Verification items for the finished model (mm, model axes). Face numbers are marked on the shaded views. A direction names the side the tool comes from. Coordinates: 2 decimals unless noted, no trailing zeros. Loops run counter-clockwise (first coordinate to the right, second up) from the corner with the lowest first, then second, coordinate; pieces in that order, holes last. Notation, with made-up numbers: (-13, 58.5) -> (-7, 58.5) arc R29 cw to (-7, 92.5) -> close; hole circle Ø3 at (41, 7.5). An arc over 180 degrees is marked (long way). Answer as a JSON object with one key per item and string values. Group by question number.
Q1. Cross-section at A-A on y = 1. Record the boundary of the cut face in (x, z).
Q2. Gauge pin test, flat ends, axial feed: pin 1 Ø2 at (x, z) = (-19.5, 1.5) entering from +Y; pin 2 Ø0.6 at (x, y) = (23.5, 1.5) entering from +Z; pin 3 Ø6 at (x, y) = (8, 9) entering from +Z; pin 4 Ø1.6 at (x, z) = (24.5, 2) entering from +Y. Record the tip position at first contact, or that the pin passes through.
Q3. Cross-section at B-B on x = -5. Record the boundary of the cut face in (y, z), and give its area (3 significant figures).
Q4. Cross-section at D-D on z = 5.5. Record the boundary of the cut face in (x, y).
Q5. Scan lines: L1, parallel to X at y = 9.5, z = 0.75; L2, parallel to Z at x = 24.5, y = 0.75; L3, parallel to X at y = 11.25, z = 1.75. Record each from-to range of solid material in increasing order.
Q6. Release check for a two-part mould opening along X. For the marked faces 1, 2, 3 and 4 record: released by +X, released by -X, zero draft, split by the parting line, or undercut.
Q7. Cross-section at C-C on z = 2.5. Record the boundary of the cut face in (x, y).
Q8. Set-up check for the marked faces 5 and 6: record each of +Z, -Z, +X, -X, +Y, -Y from which the full face is reachable in a straight line by a thin tool's end or side.
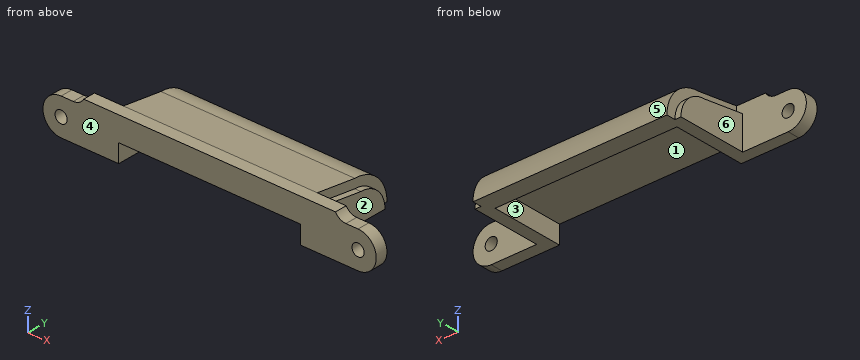
Autodesk Inventor part; units mm, degrees
ref_plane "YZ Plane" through (0, 0, 0) normal (1, 0, 0) x (0, 1, 0)
ref_plane "XZ Plane" through (0, 0, 0) normal (0, 1, 0) x (-1, 0, 0)
ref_plane "XY Plane" through (0, 0, 0) normal (0, 0, 1) x (1, 0, 0)
sketch "Sketch1" plane through (0, 0, 0) normal (0, 1, 0) x (-1, 0, 0)
  line L0 (0, 0) -> (24.5, 0)
  line L1 (24.5, 0) -> (24.5, 5)
  line L2 (24.5, 5) -> (0, 5)
  line L3 (0, 5) -> (0, 0)
  circle A0 centre (24.5, 2) radius 3
  circle A1 centre (24.5, 2) radius 1
  line L4 (0, 0) -> (15.5, 0)
  line L5 (15.5, 0) -> (15.5, 3)
  line L6 (15.5, 3) -> (0, 3)
  line L7 (0, 3) -> (0, 0)
  line L8 (0, 3) -> (6.5, 3)
  line L9 (6.5, 3) -> (6.5, 6)
  line L10 (6.5, 6) -> (0, 6)
  line L11 (0, 6) -> (0, 3)
  line L12 (6.5, 6) -> (20.5, 6)
  line L13 (20.5, 6) -> (20.5, 5)
  line L14 (20.5, 5) -> (6.5, 5)
  line L15 (6.5, 5) -> (6.5, 6)
  circle A2 centre (22.5, 7) radius 2
  line L16 (20.5, 6) -> (24.5, 6)
  line L17 (24.5, 6) -> (24.5, 5)
  line L18 (24.5, 5) -> (20.5, 5)
  line L19 (20.5, 5) -> (20.5, 6)
  line L20 (15.5, 0) -> (24.5, 0)
  line L21 (24.5, 0) -> (24.5, -1)
  line L22 (24.5, -1) -> (15.5, -1)
  line L23 (15.5, -1) -> (15.5, 0)
  point P0 (22.5, 5)
  point P1 (20.7679, 6)
  point P2 (0, 3)
  point P3 (22.2639, 0)
  point P4 (0, 5)
  dimension "d1" = 6
  dimension "d0" = 24.5
  dimension "d2" = 2
  dimension "d3" = 2
  dimension "d4" = 3
  dimension "d5" = 3
  dimension "d6" = 9
  dimension "d7" = 3
  dimension "d8" = 18
  dimension "d9" = 4
  dimension "d10" = 4
  dimension "d11" = 2
extrude "Extrusion1" add sketch "Sketch1" along normal blind 2 contours L5 L6 L9 L2 A0 L0 | L0 A0 L22 L23 | L3 L2 L9 L6 | A0 L1 A1 L0 | L0 L21 A0 | L11 L10 L9 L2 | L1 A1 A0 L21 | L9 L12 L13 L2 | L2 L13 L16 A2
sketch "Sketch2" plane through (0, 0, 6) normal (1, 0, 0) x (0, 0, -1)
  line L0 (0, 0) -> (0, 2)
  line L1 (0, 2) -> (3, 2)
  line L2 (3, 2) -> (3, 12)
  line L3 (3, 12) -> (0, 12)
  line L4 (0, 12) -> (0, 2)
  line L5 (3, 0) -> (3, 2)
  line L6 (0, 12) -> (7, 12)
  line L7 (7, 12) -> (7, 15)
  line L8 (7, 15) -> (0, 15)
  line L9 (0, 15) -> (0, 12)
  circle A0 centre (7, 9) radius 3
  line L10 (4, 9) -> (4, 0)
  line L11 (3, 0) -> (5, 0)
  line L12 (3, 0) -> (3, 12)
  circle A1 centre (7, 9) radius 6
  line L13 (0, 2) -> (1, 2)
  line L14 (0, 2) -> (1, 9)
  point P0 (6, 0)
  point P1 (3, 9)
  point P2 (4, 6.7639)
  dimension "d20" = 6
  dimension "d14" = 10
  dimension "d15" = 0
  dimension "d16" = 7
  dimension "d17" = 3
  dimension "d21" = 3
  dimension "d22" = 7
extrude "Extrusion2" add sketch "Sketch2" against normal blind 16 contours L14 A1 L2 L1 | A1 L3 L2 | L2 A1 L10 L11 L5 | A1 L7 L6 L3 | L2 L6 A0 L10 A1
sketch "Sketch3" plane through (-16, 0, 6) normal (-1, 0, 0) x (0, 0, 1)
  arc A0 (-4, 9) -> (-7, 12) centre (-7, 9) ccw
  circle A1 centre (-7, 9) radius 2
  line L0 (-7, 12) -> (-7, 9)
  line L1 (-7, 9) -> (-7, 0)
  line L2 (-7, 0) -> (-7, 2)
  circle A2 centre (-7, 9) radius 6
  line L3 (-7, 15) -> (-7, 9)
  arc A3 (-1, 9) -> (-7, 15) centre (-7, 9) ccw
  line L4 (0, 2) -> (-1, 9)
  line L5 (-1, 9) -> (0, 2)
  line L6 (-1, 2) -> (-7, 2)
  line L7 (0, 2) -> (-7, 2)
  circle A4 centre (-7, 9) radius 4.5
  line L8 (-2.5, 9) -> (-1, 9)
  line L9 (-1, 2) -> (0, 2)
  line L10 (0, 2) -> (-1.5, 2)
  line L11 (-1.5, 2) -> (-2.5, 9)
  point P0 (-6, 0)
  point P1 (-6, 2)
  point P2 (-7, 13.5)
  point P3 (-7, 12)
  point P4 (-1.5, 2)
  dimension "d23" = 4
  dimension "d24" = 9
  dimension "d25" = 1.5
extrude "Extrusion3" add sketch "Sketch3" along normal blind 1 and the other way blind 1 contours A1 L1 L0 | A1 L0 L3 A4 L1 | A4 L11 A2 L1 | A2 L11 L6 L1 picked at (-5.7494, 8.5624) picked at (-6.0599, 11.9521)
sketch "Sketch4" plane through (-15.5, 0, -1) normal (0, 0, -1) x (-1, 0, 0)
  line L0 (-0.5, 2) -> (-0.5, 9)
  line L1 (0, 0) -> (0, 2)
  line L2 (-0.5, 2) -> (0, 2)
  line L3 (0, 2) -> (0, 0)
  line L4 (0, 0) -> (-0.5, 0)
  line L5 (-0.5, 0) -> (-0.5, 2)
  point P0 (-15.5, 0)
extrude "Extrusion4" add sketch "Sketch4" against normal up to surface (3 mm away)
mirror "Mirror1" about plane through (0, 0, 6) normal (1, 0, 0) of "Extrusion1", "Extrusion2", "Extrusion3", "Extrusion4"
properties part number "battery mount rear"
Computed values:
{
 "1": {"outline": "(-24.5, -1) -> (-15, -1) -> (-15, 2) -> (15, 2) -> (15, -1) -> (24.5, -1) arc R3 ccw to (24.5, 5) -> (22.5, 5) arc R2 cw to (20.77, 6) -> (-20.77, 6) arc R2 cw to (-22.5, 5) -> (-24.5, 5) arc R3 ccw to start; hole circle Ø2 at (-24.5, 2); hole circle Ø2 at (24.5, 2)"},
 "2": {"pin 1": "stops at y = 2", "pin 2": "stops at z = 5", "pin 3": "stops at z = 5.43", "pin 4": "passes through"},
 "3": {"outline": "(0, 2) -> (9, 2) arc R3 cw to (12, -1) -> (15, -1) arc R6 ccw to (9, 5) -> (2, 6) -> (0, 6) -> close", "area": "53.7 mm²"},
 "4": {"outline": "(-21.18, 0) -> (21.18, 0) -> (21.18, 2) -> (16, 2) -> (16, 5.5) -> (-16, 5.5) -> (-16, 2) -> (-21.18, 2) -> close"},
 "5": {"L1": "x = -17 to -15, 15 to 17", "L2": "z = -1 to 1, 3 to 5", "L3": "x = -17 to 17"},
 "6": {"face 1": "undercut", "face 2": "released by +X", "face 3": "undercut", "face 4": "zero draft"},
 "7": {"outline": "(-27.46, 0) -> (-25.37, 0) -> (-25.37, 2) -> (-27.46, 2) -> close; (-23.63, 0) -> (23.63, 0) -> (23.63, 2) -> (17, 2) -> (17, 11.83) -> (16, 11.83) -> (16, 13.87) -> (-16, 13.87) -> (-16, 11.83) -> (-17, 11.83) -> (-17, 2) -> (-23.63, 2) -> close; (25.37, 0) -> (27.46, 0) -> (27.46, 2) -> (25.37, 2) -> close"},
 "8": {"face 5": "+Z, +X, -X, +Y", "face 6": "+Z, -Z, -X, +Y"}
}
